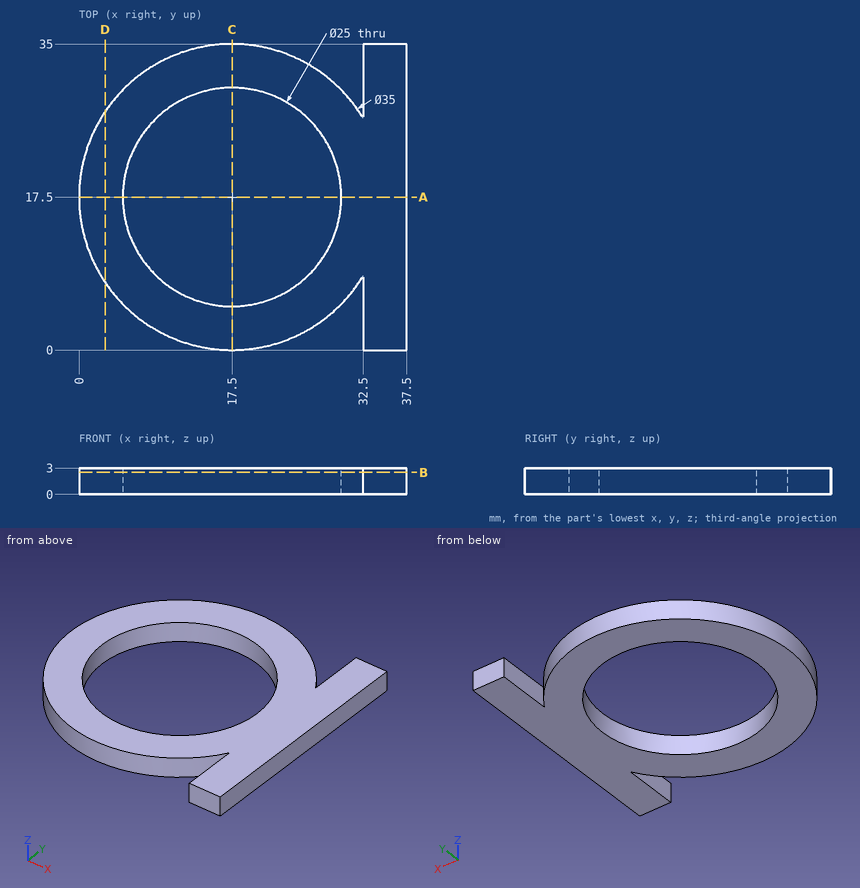
Could you check a few things on this drawing? It's one solid part, dimensions in mm from its lowest x, y, z. Coordinates: 2 decimals unless noted, no trailing zeros. Loops run counter-clockwise (first coordinate to the right, second up) from the corner with the lowest first, then second, coordinate; pieces in that order, holes last.
1. I need wall thicknesses on L1, parallel to Y at x = 17.5, z = 1.2; L2, parallel to X at y = 6.5, z = 0.9; L3, parallel to Y at x = 15.5, z = 0.4. Which ranges of each line are inside material? Lowest first, please.
2. Imagine slicing it at A-A (y = 17.5). Please give me the cut outline in (x, z).
3. For P1, Ø1.5, axis at y = 31, z = 1, coming from the -X side, with a flat end and sliding along its axis, tell me the tip position at first contact or that it passes through.
4. Imagine slicing it at D-D (x = 3). Please give me the cut outline in (y, z), and give its area (3 significant figures).
5. Imagine slicing it at C-C (x = 17.5). Please give me the cut outline in (y, z), and give its area (3 significant figures).
6. Imagine slicing it at B-B (z = 2.5). Please give me the cut outline in (x, y), and give its area (3 significant figures).
Computed values:
1. L1: y = 0 to 5, 30 to 35
1. L2: x = 3.89 to 11.56, 23.44 to 31.11, 32.5 to 37.5
1. L3: y = 0.11 to 5.16, 29.84 to 34.89
2. outline: (0, 0) - (5, 0) - (5, 3) - (0, 3) - close; (30, 0) - (37.5, 0) - (37.5, 3) - (30, 3) - close
3. P1: stops at x = 5.51
4. outline: (7.7, 0) - (27.3, 0) - (27.3, 3) - (7.7, 3) - close
4. area: 58.8 mm2
5. outline: (0, 0) - (5, 0) - (5, 3) - (0, 3) - close; (30, 0) - (35, 0) - (35, 3) - (30, 3) - close
5. area: 30.0 mm2
6. outline: (32.5, 0) - (37.5, 0) - (37.5, 35) - (32.5, 35) - (32.5, 26.51) arc R17.5 ccw (long way) to (32.5, 8.49) - close; hole circle Ø25 at (17.5, 17.5)
6. area: 616 mm2
